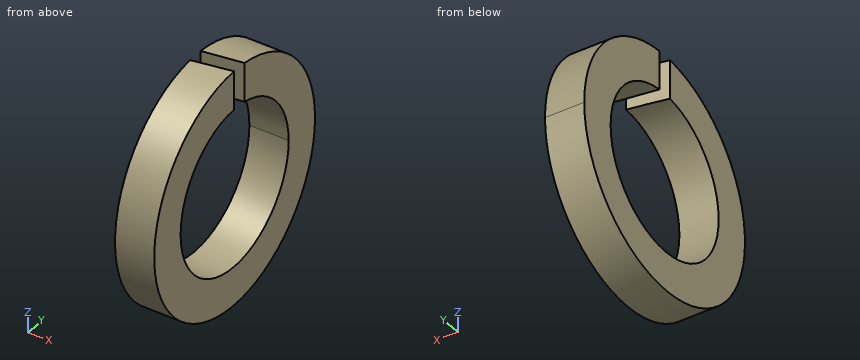
Autodesk Inventor part; units mm, degrees
ref_plane "Work Plane1" through (0, 0, 0) normal (0, -1, 0) x (1, 0, 0)
ref_plane "YZ Plane" through (0, 0, 0) normal (1, 0, 0) x (0, 1, 0)
ref_plane "XZ Plane" through (0, 0, 0) normal (0, 1, 0) x (-1, 0, 0)
sketch "Náčrt1" plane through (0, 0, 0) normal (1, 0, 0) x (0, 1, 0)
  circle A0 centre (0, 0) radius 6.1
  circle A1 centre (0, 0) radius 4.1
  dimension "d0" = 8.2
  dimension "d1" = 12.2
extrude "Těleso" add sketch "Náčrt1" along normal blind 2
sketch "Náčrt2" plane through (0, 0, 0) normal (0, 0, 1) x (1, 0, 0)
  line L0 (0, -4.1) -> (0, 4.1)
  line L1 (2, 6.1) -> (2, -6.1)
  line L2 (-1.2, 0) -> (7.2, 0)
  line L3 (0, -0.4) -> (2, -0.0473)
  line L4 (0, 0.4) -> (2, 0.7527)
  dimension "d4" = 0.4
  dimension "d5" = 0.4
  dimension "d6" = 80
extrude "Výřez" cut sketch "Náčrt2" along normal up to next
ref_plane "Work Plane1" through (0, 0, 0) normal (0, -1, 0) x (1, 0, 0)
equation "\"d0\" = SD1"
equation "\"d1\" = SD2"
equation "\"d2\" = SD"
equation "\"d4\" = 0.2 * SD"
equation "\"d5\" = 0.2 * SD"
equation "\"d6\" = FAWI"
equation "\"d7\" = SD"
equation "\"SD1\" = 8.2"
equation "\"SD2\" = 12.2"
equation "\"SD\" = 2"
equation "\"FAWI\" = 80deg"
equation "\"NND\" = 8"
properties part number "CSN 02 1740 - 8" material "Nerezová ocel"
Verification items for the finished model (mm, model axes). Coordinates: 2 decimals unless noted, no trailing zeros. Loops run counter-clockwise (first coordinate to the right, second up) from the corner with the lowest first, then second, coordinate; pieces in that order, holes last. Notation, with made-up numbers: (53.25, -23) - (104.25, -23) arc R21 cw to (104.25, 2) - close; hole circle Ø1 at (-39.75, 59.5). An arc over 180 degrees is marked (long way). Put each result on its own line as item: value.
Item 1: Section check A-A (z = 5.25). Enter the section's corners in (x, y), then the cut area to 3 significant figures.
Conclusion:
outline: (0, -3.11) - (2, -3.11) - (2, -0.05) - (0, -0.4) - close; (0, 0.4) - (2, 0.75) - (2, 3.11) - (0, 3.11) - close
area: 10.8 mm2
Item 2: Section check C-C (x = 0.35). Enter the section's corners in (y, z).
Conclusion:
outline: (-0.34, 4.09) - (-0.34, 6.09) arc R6.1 ccw (long way) to (0.46, 6.08) - (0.46, 4.07) arc R4.1 cw (long way) to start
Item 3: Section check B-B (y = 2.5). Enter the section's corners in (x, z), then the cut area to 3 significant figures.
Conclusion:
outline: (0, -5.56) - (2, -5.56) - (2, -3.25) - (0, -3.25) - close; (0, 3.25) - (2, 3.25) - (2, 5.56) - (0, 5.56) - close
area: 9.26 mm2
Item 4: Scan lines: line 1 along Y through (x, z) = (0.95, 0); line 2 along Z through (x, y) = (0.5, 0); line 3 along Z through (x, y) = (0.2, 2.75). Record each from-to range of solid material in increasing order.
Conclusion:
line 1: y = -6.1 to -4.1, 4.1 to 6.1
line 2: z = -6.1 to -4.1
line 3: z = -5.44 to -3.04, 3.04 to 5.44
